Autodesk Inventor part; units mm, degrees
ref_plane "YZ Plane" through (0, 0, 0) normal (1, 0, 0) x (0, 1, 0)
ref_plane "XZ Plane" through (0, 0, 0) normal (0, 1, 0) x (-1, 0, 0)
ref_plane "XY Plane" through (0, 0, 0) normal (0, 0, 1) x (1, 0, 0)
sketch "Sketch1" plane through (0, 0, 0) normal (0, 1, 0) x (-1, 0, 0)
  line L0 (0, 0) -> (0, -6)
  line L1 (0, -6) -> (4, -6)
  line L2 (4, -6) -> (4, -50)
  line L3 (4, -50) -> (0, -50)
  line L4 (0, -50) -> (0, -56)
  line L5 (0, 0) -> (10, 0)
  line L6 (0, 0) -> (10, 0)
  line L7 (10, 0) -> (10, -11.5)
  line L8 (10, -11.5) -> (18, -11.5)
  line L9 (18, -11.5) -> (18, -16.5)
  line L10 (18, -16.5) -> (10, -16.5)
  line L11 (10, -16.5) -> (10, -63)
  line L12 (10, -63) -> (18, -63)
  line L13 (18, -63) -> (18, -68)
  line L14 (18, -68) -> (10, -68)
  line L15 (0, -56) -> (4, -56)
  line L16 (4, -56) -> (4, -68)
  line L17 (4, -68) -> (10, -68)
  point P0 (0, -3)
  point P1 (0, -53)
  dimension "d2" = 50
  dimension "d3" = 6
  dimension "d4" = 4
  dimension "d19" = 6
  dimension "d20" = 11.5
  dimension "d21" = 5
  dimension "d22" = 8
  dimension "d23" = 46.5
extrude "Extrusion1" add sketch "Sketch1" along normal blind 6
sketch "Sketch4" plane through (0, 0, -50) normal (1, 0, 0) x (0, 0, -1)
  line L0 (-44, 0) -> (0, 0)
  line L1 (-50, 0) -> (-50, 6)
  line L2 (-44, 0) -> (-50, 6) construction
  circle A0 centre (-47, 3) radius 1.75
  line L3 (0, 0) -> (6, 0)
  line L4 (-44, 6) -> (0, 6)
  line L5 (6, 0) -> (0, 6) construction
  circle A1 centre (3, 3) radius 1.75
  dimension "d24" = 3.5
extrude "Extrusion4" cut sketch "Sketch4" against normal through all
chamfer "Chamfer2" distance 1 angle 45 8 edges at (-5, 6, 0) (-2, 6, -6) (-2, 0, -6) (-5, 0, 0) (-2, 0, -50) (-2, 6, -50) (-2, 0, -56) (-2, 6, -56)
chamfer "Chamfer3" distance 2 angle 45 1 edges at (-4, 3, -68)
sketch "Sketch5" plane through (-18, 0, -11.5) normal (0, 0, 1) x (1, 0, 0)
  circle A0 centre (3, 3) radius 3 construction
  line L0 (0, 6) -> (8, 6)
  line L1 (0, 0) -> (0, 6)
  line L2 (0, 0) -> (8, 0)
  circle A1 centre (3, 3) radius 1.75
  point P0 (18, 0)
  dimension "d33" = 3.5
chamfer "Chamfer4" distance 1 angle 45 4 edges at (-18, 0, -65.5) (-18, 6, -65.5) (-18, 0, -14) (-18, 6, -14)
extrude "Extrusion5" cut sketch "Sketch5" against normal through all
chamfer "Chamfer5" distance 1 angle 45 2 edges at (-16.75, 3, -11.5) (-16.75, 3, -68)
properties part number "camadapter2"
Design review of the part built by this model. Coordinates are the model's own, in mm. A direction names the side the tool comes from. Give positions to 0.01 mm unless a question says otherwise; leave off trailing zeros. Write each loop counter-clockwise with the first axis right and the second up, starting at its lowest first coordinate (ties: lowest second). Pieces come first, ordered by that corner, then holes. Notation, with made-up numbers: (18.25, 76.5) - (24.25, 76.5) arc R34 ccw to (24.25, 110.5) - close; hole circle Ø11 at (21.25, 58.25). An arc over 180 degrees is marked (long way). Return JSON: item names as keys, results as strings. Group by question number.
(1) We need section B-B, the plane z = -3. Give the boundary of the cut face in (x, y), then the cut area to 3 significant figures.
(2) Insertion check: pin 1 (1.2 mm diameter, centred on x = -2, y = 2.5, fed in from -Z); pin 2 (3 mm diameter, centred on x = -12.5, y = 2, fed in from +Z); pin 3 (3 mm diameter, centred on y = 4.5, z = -34.5, fed in from +X). Each pin has a flat end and moves straight along its axis. Give the tip position at first contact, or say it passes through.
(3) We need section D-D, the plane x = -5. Give the boundary of the cut face in (y, z), then the cut area to 3 significant figures.
(4) We need section A-A, the plane x = -10.75. Give the boundary of the cut face in (y, z).
(5) To check wall thickness, follow probe 1 along Y at (x, z) = (-15, -14.05); probe 2 along Z at (x, y) = (-0.75, 3.75); probe 3 along Z at (x, y) = (-5, 4). State the ranges of each line that lie inside material, in increasing order.
(6) Machinability: for faces 1 (the flat face through (-2, 3, -50)), 2 (the flat face through (-12, 3, -11.5)), 3 (the flat face through (-10, 3, -39)), which of the approach directions +Z, -Z, +X, -X, +Y, -Y give a long, thin tool a straight path to every point of the face, cutting with its end or side? Answer none if there is none.
(7) Mouldability with a two-part tool opening along Z and no side actions: class faces 4 (the cylindrical face through (-4.93, 1.45, -3.81)), 5 (the flat face through (-2, 3, -56)), 6 (the flat face through (-8, 6, -34)) as +Z half, -Z half, draft (parallel to the pull), parting line (faces both ways), or undercut.
(8) We need section C-C, the plane x = -15. Give the boundary of the cut face in (y, z).
Reported:
{
 "1": {"outline": "(-10, 0) - (0, 0) - (0, 1.25) - (-10, 1.25) - close; (-10, 4.75) - (0, 4.75) - (0, 6) - (-10, 6) - close", "area": "25.0 mm2"},
 "2": {"pin 1": "stops at z = -56", "pin 2": "stops at z = -11.5", "pin 3": "stops at x = -4"},
 "3": {"outline": "(0, -67) - (6, -67) - (6, -1) - (5, 0) - (1, 0) - (0, -1) - close; hole circle Ø3.5 at (3, -53); hole circle Ø3.5 at (3, -3)", "area": "382 mm2"},
 "4": {"outline": "(0, -68) - (6, -68) - (6, -63) - (0, -63) - close; (0, -16.5) - (6, -16.5) - (6, -11.5) - (0, -11.5) - close"},
 "5": {"probe 1": "y = 0 to 1.25, 4.75 to 6", "probe 2": "z = -56 to -54.58, -51.42 to -50, -6 to -4.58, -1.42 to 0", "probe 3": "z = -67 to -54.44, -51.56 to -4.44, -1.56 to 0"},
 "6": {"face 1": "+X, +Y, -Y", "face 2": "+Z, -X, +Y, -Y", "face 3": "-X, +Y, -Y"},
 "7": {"face 4": "undercut", "face 5": "-Z half", "face 6": "draft"},
 "8": {"outline": "(0, -68) - (0.25, -68) - (1.25, -67) - (1.25, -63) - (0, -63) - close; (0, -16.5) - (1.25, -16.5) - (1.25, -12.5) - (0.25, -11.5) - (0, -11.5) - close; (4.75, -67) - (5.75, -68) - (6, -68) - (6, -63) - (4.75, -63) - close; (4.75, -16.5) - (6, -16.5) - (6, -11.5) - (5.75, -11.5) - (4.75, -12.5) - close"}
}
